The listing builds one solid part. Answer for the finished solid, in the listing's coordinates (mm). Face numbers are marked on the shaded views. A direction names the side the tool comes from. Give positions to 0.01 mm unless a question says otherwise; leave off trailing zeros. Order: outer loops, then holes, each group sorted by start corner. A loop starts at its lowest first (then second) coordinate and runs counter-clockwise, first axis right, second up.
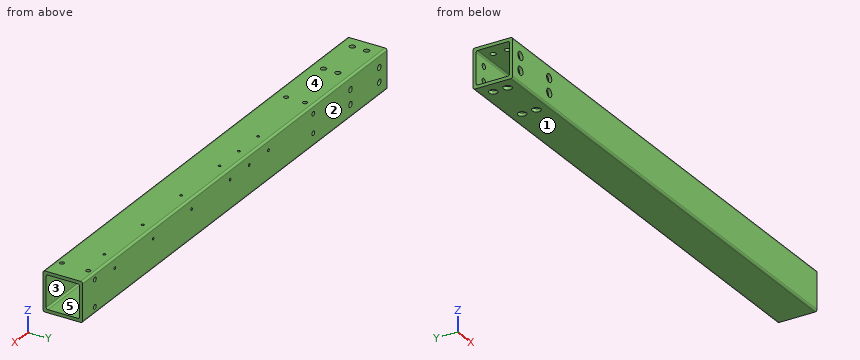
```python
from build123d import *

# Parameters (mm, degrees)
BOSS_EXTRUDE1_DEPTH                  = 237.5
BOSS_EXTRUDE1_DEPTH_BACK             = 237.5
TAP_DRILL_FOR_M5X0_8_TAP1_D          = 4.2
TAP_DRILL_FOR_M5X0_8_TAP1_DEPTH      = 3.048
TAP_DRILL_FOR_M3X0_5_TAP1_D          = 2.5
TAP_DRILL_FOR_M3X0_5_TAP1_DEPTH      = 3.048
TAP_DRILL_FOR_M5X0_8_TAP2_AT_2_COUNT = 2
TAP_DRILL_FOR_M5X0_8_TAP2_AT_2_PITCH = 25.4
M5_CLEARANCE_HOLE1_D                 = 5.3
M5_CLEARANCE_HOLE1_DEPTH             = 3.048
F_8_0_8_DIAMETER_HOLE1_D             = 8
F_8_0_8_DIAMETER_HOLE1_DEPTH         = 3.048
F_8_0_8_DIAMETER_HOLE2_D             = 8
F_8_0_8_DIAMETER_HOLE2_DEPTH         = 3.048


with BuildPart() as part:
    # Sketch4 → Boss-Extrude1 (new, two sides: drawn at the far end of the back side and taken through both)
    with BuildSketch(Plane(origin=(0, 0, 0), x_dir=(0, 0, -1), z_dir=(1, 0, 0)).offset(-BOSS_EXTRUDE1_DEPTH_BACK)):
        with BuildLine():
            Line((19.05, -17.145), (19.05, 17.145))
            ThreePointArc((19.05, 17.145), (18.492038418, 18.492038418), (17.145, 19.05))
            Line((17.145, 19.05), (-17.145, 19.05))
            ThreePointArc((-17.145, 19.05), (-18.492038418, 18.492038418), (-19.05, 17.145))
            Line((-19.05, 17.145), (-19.05, -17.145))
            ThreePointArc((-19.05, -17.145), (-18.492038418, -18.492038418), (-17.145, -19.05))
            Line((-17.145, -19.05), (17.145, -19.05))
            ThreePointArc((17.145, -19.05), (18.492038418, -18.492038418), (19.05, -17.145))
        make_face()
        with BuildLine():
            Line((16.002, 14.4018), (16.002, -14.4018))
            ThreePointArc((16.002, -14.4018), (15.533312271, -15.533312271), (14.4018, -16.002))
            Line((14.4018, -16.002), (-14.4018, -16.002))
            ThreePointArc((-14.4018, -16.002), (-15.533312271, -15.533312271), (-16.002, -14.4018))
            Line((-16.002, -14.4018), (-16.002, 14.4018))
            ThreePointArc((-16.002, 14.4018), (-15.533312271, 15.533312271), (-14.4018, 16.002))
            Line((-14.4018, 16.002), (14.4018, 16.002))
            ThreePointArc((14.4018, 16.002), (15.533312271, 15.533312271), (16.002, 14.4018))
        make_face(mode=Mode.SUBTRACT)
    extrude(amount=BOSS_EXTRUDE1_DEPTH + BOSS_EXTRUDE1_DEPTH_BACK)

    # Tap Drill for M5x0.8 Tap1
    with Locations(Plane(origin=(0, 19.05, 0), x_dir=(1, 0, 0), z_dir=(0, 1, 0))):
        with Locations((-122.5, 7.05), (-122.5, -10.95)):
            tap_drill_for_m5x0_8_tap1 = Hole(TAP_DRILL_FOR_M5X0_8_TAP1_D / 2, depth=TAP_DRILL_FOR_M5X0_8_TAP1_DEPTH)

    # Tap Drill for M3x0.5 Tap1
    with Locations(Plane.XY.offset(19.05)):
        with Locations((187.5, 9.05), (127.5, 9.05), (67.5, 9.05), (7.5, 9.05), (-52.5, 9.05), (-22.5, 9.05)):
            tap_drill_for_m3x0_5_tap1 = Hole(TAP_DRILL_FOR_M3X0_5_TAP1_D / 2, depth=TAP_DRILL_FOR_M3X0_5_TAP1_DEPTH)

    # Sketch22 → Tap Drill for M5x0.8 Tap2 (revolve, cut)
    with BuildSketch(Plane(origin=(218.45, 12.7, 19.05), x_dir=(0, -1, 0), z_dir=(1, 0, 0))):
        Polygon((0, 0), (0, 6.2618073), (2.1, 5), (2.1, 0), align=None)
    tap_drill_for_m5x0_8_tap2 = revolve(axis=Axis((218.45, 12.7, 25.4), (0, 0, -1)), mode=Mode.SUBTRACT)

    # Tap Drill for M5x0.8 Tap2 at 2: Tap Drill for M5x0.8 Tap2 ×2
    with Locations(*[(0, -i * TAP_DRILL_FOR_M5X0_8_TAP2_AT_2_PITCH, 0) for i in range(1, TAP_DRILL_FOR_M5X0_8_TAP2_AT_2_COUNT)]):
        add(tap_drill_for_m5x0_8_tap2, mode=Mode.SUBTRACT)

    # Mirror1: Tap Drill for M5x0.8 Tap1, Tap Drill for M3x0.5 Tap1, Tap Drill for M5x0.8 Tap2 across plane
    add(tap_drill_for_m5x0_8_tap1.mirror(Plane(origin=(0, 0, 0), x_dir=(0, 0.7071067811865478, 0.7071067811865472), z_dir=(0, -0.7071067811865475, 0.7071067811865477))), mode=Mode.SUBTRACT)
    add(tap_drill_for_m3x0_5_tap1.mirror(Plane(origin=(0, 0, 0), x_dir=(0, 0.7071067811865478, 0.7071067811865472), z_dir=(0, -0.7071067811865475, 0.7071067811865477))), mode=Mode.SUBTRACT)
    add(tap_drill_for_m5x0_8_tap2.mirror(Plane(origin=(0, 0, 0), x_dir=(0, 0.7071067811865478, 0.7071067811865472), z_dir=(0, -0.7071067811865475, 0.7071067811865477))), mode=Mode.SUBTRACT)

    # Mirror1 copy 1 sketch → Mirror1 copy 1 (revolve, cut)
    with BuildSketch(Plane(origin=(218.45, 19.05, -12.7), x_dir=(0, 0, -1), z_dir=(1, 0, 0))):
        Polygon((0, 0), (0, -6.2618073), (2.1, -5), (2.1, 0), align=None)
    revolve(axis=Axis((218.45, 25.4, -12.7), (0, 1, 0)), mode=Mode.SUBTRACT)

    # M5 Clearance Hole1
    with Locations(Plane(origin=(0, 19.05, 0), x_dir=(1, 0, 0), z_dir=(0, 1, 0))):
        with Locations((-225.5, 6.8), (-225.5, -6.95), (-180.5, -6.95), (-180.5, 6.8)):
            m5_clearance_hole1 = Hole(M5_CLEARANCE_HOLE1_D / 2, depth=M5_CLEARANCE_HOLE1_DEPTH)

    # Mirror2: M5 Clearance Hole1 across plane
    add(m5_clearance_hole1.mirror(Plane(origin=(0, 0, 0), x_dir=(0, 0.7071067811865478, 0.7071067811865472), z_dir=(0, -0.7071067811865475, 0.7071067811865477))), mode=Mode.SUBTRACT)

    # Ø8.0 (8) Diameter Hole1
    with Locations(Plane.XY.offset(-16.002)):
        with Locations((-225.5, -6.8), (-225.5, 6.95), (-180.5, 6.95), (-180.5, -6.8)):
            Hole(F_8_0_8_DIAMETER_HOLE1_D / 2, depth=F_8_0_8_DIAMETER_HOLE1_DEPTH)

    # Ø8.0 (8) Diameter Hole2
    with Locations(Plane(origin=(0, -16.002, 0), x_dir=(1, 0, 0), z_dir=(0, 1, 0))):
        with Locations((-225.5, 6.8), (-225.5, -6.95), (-180.5, -6.95), (-180.5, 6.8)):
            Hole(F_8_0_8_DIAMETER_HOLE2_D / 2, depth=F_8_0_8_DIAMETER_HOLE2_DEPTH)


solid = part.part
```
1) Find section A-A (x = -58). Write down the section's boundary in (y, z) (3 decimals), then the cut area to 3 significant figures.
Geometry says:
outline: (-19.05, -17.145) arc R1.905 ccw to (-17.145, -19.05) - (17.145, -19.05) arc R1.905 ccw to (19.05, -17.145) - (19.05, 17.145) arc R1.905 ccw to (17.145, 19.05) - (-17.145, 19.05) arc R1.905 ccw to (-19.05, 17.145) - close; hole (-16.002, -14.402) arc R1.6 ccw to (-14.402, -16.002) - (14.402, -16.002) arc R1.6 ccw to (16.002, -14.402) - (16.002, 14.402) arc R1.6 ccw to (14.402, 16.002) - (-14.402, 16.002) arc R1.6 ccw to (-16.002, 14.402) - close
area: 426 mm2
2) A tool of negligible diameter and unlimited length cuts with its end or side. For the marked faces 4 and 5, from which of +Z, -Z, +X, -X, +Y, -Y can it reach the whole face along a straight path? Write none if from no direction.
Geometry says:
face 4: +Z, +X, -X, +Y, -Y
face 5: +X, -X
3) For a pull along Y with two mould halves and no side action, classify the marked faces 1, 2 and 3 as +Y half, -Y half, draft (parallel to the pull), parting line (faces both ways), or undercut.
Geometry says:
face 1: draft
face 2: +Y half
face 3: undercut
4) Given P1, Ø4, axis at x = 218.45, z = -12.7, coming from the +Y side; P2, Ø7, axis at x = -180.5, y = 6.95, coming from the -Z side, each flat-ended and moving along its own axis, determine where each tip first touches the part or whether it passes through.
Geometry says:
P1: stops at y = -15.97
P2: stops at z = 16
5) Straight lines are drawn through the part: probe 1 along Y at (x, z) = (29, 8); probe 2 along Y at (x, z) = (-180.5, -17.35). For each, find the intervals that lie inside material, in ascending order.
Geometry says:
probe 1: y = -19.05 to -16, 16 to 19.05
probe 2: y = -19.04 to -10.8, -2.8 to 2.95, 10.95 to 19.04
